Source: three-view drawing plus pictorial views. Frame: mm from the lowest corner of the part. A direction names the side the tool comes from. Coordinates: 2 decimals unless noted, no trailing zeros. Write each loop counter-clockwise with the first axis right and the second up, starting at its lowest first coordinate (ties: lowest second). Pieces come first, ordered by that corner, then holes. Notation, with made-up numbers: (79, 61) -> (103, 61) arc R36 cw to (103, 95) -> close; hole circle Ø3 at (79.25, 2.25). An arc over 180 degrees is marked (long way). One line per item, written item: value.
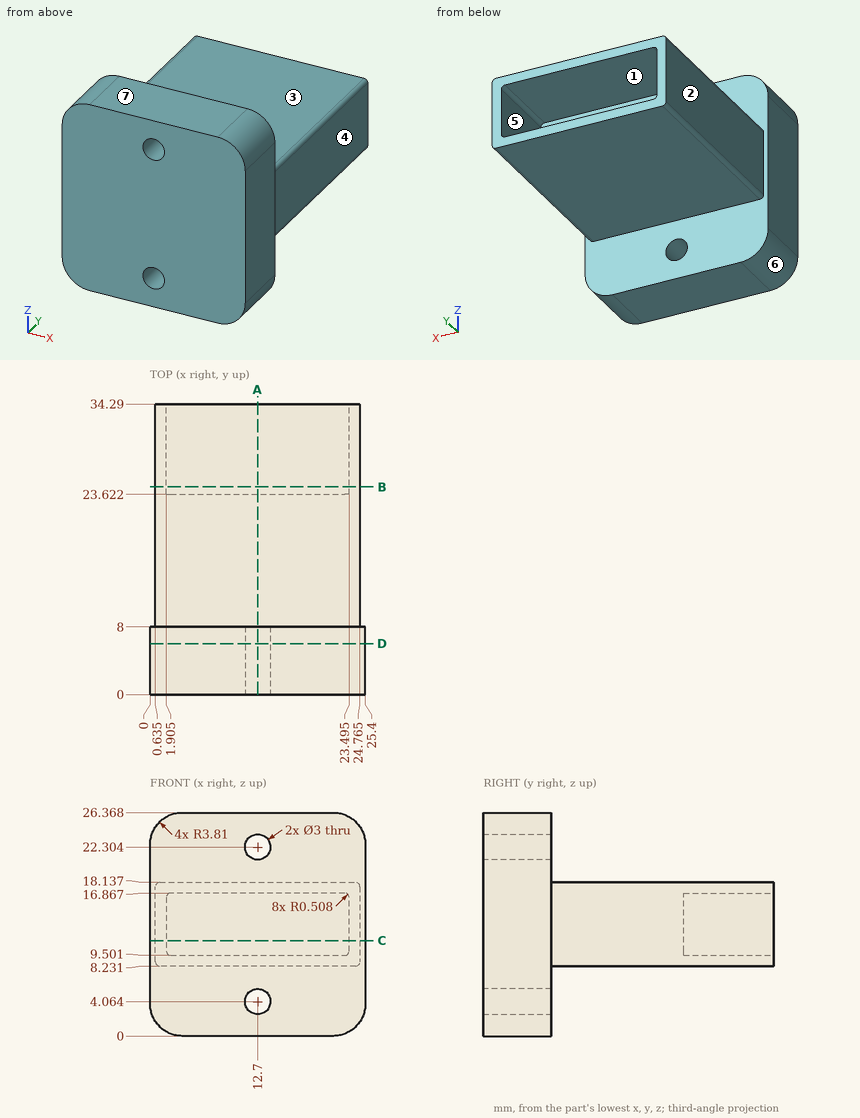
(1) First-contact query: pin 1 (3 mm diameter, centred on x = 15.5, y = 27.5, fed in from -Z); pin 2 (11.5 mm diameter, centred on x = 17.5, y = 29, fed in from +Z); pin 3 (2.5 mm diameter, centred on x = 12.7, z = 22.304, fed in from -Y); pin 4 (8 mm diameter, centred on y = 22, z = 17.5, fed in from -X) (3 decimals). Flat tips, straight axial feed; report the tip coordinate or a pass-through.
Responses:
pin 1: stops at z = 8.23
pin 2: stops at z = 18.14
pin 3: passes through
pin 4: stops at x = 0.635
(2) Section B-B (y = 24.5). Return the cut outline in (x, z) (3 decimals), then the cut area to 3 significant figures.
Responses:
outline: (0.635, 8.739) arc R0.508 ccw to (1.143, 8.231) -> (24.257, 8.231) arc R0.508 ccw to (24.765, 8.739) -> (24.765, 17.629) arc R0.508 ccw to (24.257, 18.137) -> (1.143, 18.137) arc R0.508 ccw to (0.635, 17.629) -> close; hole (1.905, 10.009) arc R0.508 ccw to (2.413, 9.501) -> (22.987, 9.501) arc R0.508 ccw to (23.495, 10.009) -> (23.495, 16.359) arc R0.508 ccw to (22.987, 16.867) -> (2.413, 16.867) arc R0.508 ccw to (1.905, 16.359) -> close
area: 80.0 mm2
(3) Section C-C (z = 11.25). Return the cut outline in (x, y) (3 decimals), then the cut area to 3 significant figures.
Responses:
outline: (0, 0) -> (25.4, 0) -> (25.4, 8) -> (24.765, 8) -> (24.765, 34.29) -> (23.495, 34.29) -> (23.495, 23.622) -> (1.905, 23.622) -> (1.905, 34.29) -> (0.635, 34.29) -> (0.635, 8) -> (0, 8) -> close
area: 607 mm2
(4) Pull-direction query (Z, two-part tool) for the marked faces 5, 6 and 7; classes: released by +Z, released by -Z, zero draft, split by the parting line, or undercut.
Responses:
face 5: undercut
face 6: released by -Z
face 7: released by +Z
(5) Section A-A (x = 12.7). Return the cut outline in (y, z), then the cut area to 3 significant figures.
Responses:
outline: (0, 0) -> (8, 0) -> (8, 2.56) -> (0, 2.56) -> close; (0, 5.56) -> (8, 5.56) -> (8, 8.23) -> (34.29, 8.23) -> (34.29, 9.5) -> (23.62, 9.5) -> (23.62, 16.87) -> (34.29, 16.87) -> (34.29, 18.14) -> (8, 18.14) -> (8, 20.8) -> (0, 20.8) -> close; (0, 23.8) -> (8, 23.8) -> (8, 26.37) -> (0, 26.37) -> close
area: 345 mm2
(6) Reachability of the marked faces 1, 2, 3 and 4 from +Z, -Z, +X, -X, +Y, -Y: full face, straight path, thin tool, end or side. Return the list, or none.
Responses:
face 1: +Y
face 2: +Z, -Z, -X, +Y
face 3: +Z, +X, -X, +Y
face 4: +Z, -Z, +X, +Y
(7) Line query: line 1 (Z direction, x = 15.5, y = 30.5); line 2 (X direction, y = 33, z = 14.25) (3 decimals); line 3 (Y direction, x = 23, z = 25). Output: solid intervals per line, ascending. Write a range as [from, to].
Responses:
line 1: z = [8.23, 9.5], [16.87, 18.14]
line 2: x = [0.635, 1.905], [23.495, 24.765]
line 3: y = [0, 8]
(8) Section D-D (y = 6). Return the cut outline in (x, z).
Responses:
outline: (0, 3.81) arc R3.81 ccw to (3.81, 0) -> (21.59, 0) arc R3.81 ccw to (25.4, 3.81) -> (25.4, 22.56) arc R3.81 ccw to (21.59, 26.37) -> (3.81, 26.37) arc R3.81 ccw to (0, 22.56) -> close; hole circle Ø3 at (12.7, 4.06); hole circle Ø3 at (12.7, 22.3)
